```python
from build123d import *

# Parameters (mm, degrees)
SKETCH1_W           = 63.5
SKETCH1_H           = 50.8
BOSS_EXTRUDE1_DEPTH = 25.2
SKETCH2_R           = 13.1445
SKETCH2_R_2         = 6.7945
BOSS_EXTRUDE2_DEPTH = 2.2
SKETCH3_R           = 2
CUT_EXTRUDE1_DEPTH  = 5.5
SKETCH4_R           = 2
CUT_EXTRUDE2_DEPTH  = 5.5
CUT_EXTRUDE3_START  = -5.5
SKETCH5_R           = 2
CUT_EXTRUDE3_DEPTH  = 5.5
FILLET1_R           = 2
SKETCH6_W           = 18
SKETCH6_H           = 12
BOSS_EXTRUDE3_DEPTH = 1


with BuildPart() as part:
    # Sketch1 → Boss-Extrude1 (new body)
    with BuildSketch(Plane(origin=(0, 0, 0), x_dir=(1, 0, 0), z_dir=(0, 1, 0))):
        Rectangle(SKETCH1_W, SKETCH1_H)
    extrude(amount=BOSS_EXTRUDE1_DEPTH)

    # Sketch2 → Boss-Extrude2 (add)
    with BuildSketch(Plane(origin=(0, 25.2, 0), x_dir=(1, 0, 0), z_dir=(0, 1, 0))):
        with Locations(Location((15.25, 0, 0), (0, 0, 90))):
            Circle(SKETCH2_R)
        with Locations(Location((15.25, 0, 0), (0, 0, 270))):
            Circle(SKETCH2_R_2, mode=Mode.SUBTRACT)
    extrude(amount=BOSS_EXTRUDE2_DEPTH)

    # Sketch3 → Cut-Extrude1 (cut)
    with BuildSketch(Plane.XY.offset(25.4)):
        with Locations((15.25, 12.6)):
            Circle(SKETCH3_R)
    extrude(amount=-CUT_EXTRUDE1_DEPTH, mode=Mode.SUBTRACT)

    # Sketch4 → Cut-Extrude2 (cut)
    with BuildSketch(Plane(origin=(31.75, 0, 0), x_dir=(0, 0, -1), z_dir=(1, 0, 0))):
        with Locations((0, 12.6)):
            Circle(SKETCH4_R)
    extrude(amount=-CUT_EXTRUDE2_DEPTH, mode=Mode.SUBTRACT)

    # Sketch5 → Cut-Extrude3 (cut)
    with BuildSketch(Plane(origin=(0, 0, -25.4), x_dir=(-1, 0, 0), z_dir=(0, 0, -1)).offset(CUT_EXTRUDE3_START)):
        with Locations(Location((-15.25, 12.6, 0), (0, 0, 180))):
            Circle(SKETCH5_R)
    extrude(amount=CUT_EXTRUDE3_DEPTH, mode=Mode.SUBTRACT)

    # Fillet1
    fillet1_edges = [part.edges().sort_by_distance(p)[0] for p in [
        (-31.75, 25.2, 0),
        (0, 25.2, 25.4),
        (31.75, 25.2, 0),
        (0, 0, 25.4),
        (-31.75, 0, 0),
        (0, 0, -25.4),
        (31.75, 0, 0),
        (0, 25.2, -25.4),
        (31.75, 12.6, 25.4),
        (-31.75, 12.6, 25.4),
        (-31.75, 12.6, -25.4),
        (31.75, 12.6, -25.4),
    ]]
    fillet(fillet1_edges, radius=FILLET1_R)

    # Sketch6 → Boss-Extrude3 (add)
    with BuildSketch(Plane(origin=(0, 0, -25.4), x_dir=(-1, 0, 0), z_dir=(0, 0, -1))):
        with Locations((16.25, 8.5)):
            Rectangle(SKETCH6_W, SKETCH6_H)
    extrude(amount=BOSS_EXTRUDE3_DEPTH)


solid = part.part
```
Part model, mm, in its own coordinate system. A direction names the side the tool comes from. Coordinates: 2 decimals unless noted, no trailing zeros. Order: outer loops, then holes, each group sorted by start corner. A loop starts at its lowest first (then second) coordinate and runs counter-clockwise, first axis right, second up. Notation, with made-up numbers: (-23.5, -31.5) - (10.5, -31.5) arc R11 cw to (10.5, -27.5) - close; hole circle Ø6 at (64, 25). An arc over 180 degrees is marked (long way). Return JSON: item names as keys, results as strings. Group by question number.
Item 1: Cut at D-D (x = -12). List the corners of the cut face in (y, z).
Item 2: Pull direction Y, two halves, no side cores. Call faces 1 (the face through (31.15, 12.75, 24.83)), 2 (the face through (0.42, 0.6, 24.83)), 3 (the face through (14.99, 14.583, 22.688)): pulls with the +Y half, pulls with the -Y half, needs draft (parallel to the pull), parting line crosses it, or undercut.
Item 3: Which spindle directions (+Z, -Z, +X, -X, +Y, -Y) get a long thin tool onto all of the face, cutting with end or side? Do faces 4 (the face through (15, 13, 19.9)), 5 (the face through (2.217, 26.285, 1.711)), 6 (the face through (15, 13, -19.9)). Say none if no direction does.
Item 4: Cut at B-B (y = 12.6). List the corners of the cut face in (x, z).
Item 5: Cut at C-C (z = 14). List the corners of the cut face in (x, y).
Item 6: Cut at A-A (z = -21). List the corners of the cut face in (x, y).
Item 7: Pin check, flat tips, straight feed: pin 1 (4 mm diameter, centred on x = -4.5, y = 22.5, fed in from -Z); pin 2 (0.5 mm diameter, centred on x = -20, z = -26, fed in from -Y); pin 3 (1.1 mm diameter, centred on y = 7, z = -26, fed in from -X). Stop position of each tip, or through.
Item 8: Drill centre lines: probe 1 along Y at (x, z) = (15, -21); probe 2 along X at (y, z) = (26, 0); probe 3 along Y at (x, z) = (-27, 1.5). Where is each one in solid material? Low to high. Write a range as from..to.
Check values:
{
 "1": {"outline": "(0, -23.4) arc R2 ccw to (2, -25.4) - (2.5, -25.4) - (2.5, -26.4) - (14.5, -26.4) - (14.5, -25.4) - (23.2, -25.4) arc R2 ccw to (25.2, -23.4) - (25.2, 23.4) arc R2 ccw to (23.2, 25.4) - (2, 25.4) arc R2 ccw to (0, 23.4) - close"},
 "2": {"face 1": "needs draft", "face 2": "pulls with the -Y half", "face 3": "undercut"},
 "3": {"face 4": "+Z", "face 5": "+Y", "face 6": "-Z"},
 "4": {"outline": "(-31.75, -23.4) arc R2 ccw to (-29.75, -25.4) - (-25.25, -25.4) - (-25.25, -26.4) - (-7.25, -26.4) - (-7.25, -25.4) - (13.25, -25.4) - (13.25, -19.9) - (17.25, -19.9) - (17.25, -25.4) - (29.75, -25.4) arc R2 ccw to (31.75, -23.4) - (31.75, -2) - (26.25, -2) - (26.25, 2) - (31.75, 2) - (31.75, 23.4) arc R2 ccw to (29.75, 25.4) - (17.25, 25.4) - (17.25, 19.9) - (13.25, 19.9) - (13.25, 25.4) - (-29.75, 25.4) arc R2 ccw to (-31.75, 23.4) - close"},
 "5": {"outline": "(-31.75, 2) arc R2 ccw to (-29.75, 0) - (29.75, 0) arc R2 ccw to (31.75, 2) - (31.75, 23.2) arc R2 ccw to (29.75, 25.2) - (-29.75, 25.2) arc R2 ccw to (-31.75, 23.2) - close"},
 "6": {"outline": "(-31.75, 2) arc R2 ccw to (-29.75, 0) - (29.75, 0) arc R2 ccw to (31.75, 2) - (31.75, 23.2) arc R2 ccw to (29.75, 25.2) - (-29.75, 25.2) arc R2 ccw to (-31.75, 23.2) - close; hole circle Ø4 at (15.25, 12.6)"},
 "7": {"pin 1": "stops at z = -25.4", "pin 2": "stops at y = 2.5", "pin 3": "stops at x = -25.25"},
 "8": {"probe 1": "y = 0..10.62, 14.58..25.2", "probe 2": "x = 2.11..8.46, 22.04..28.39", "probe 3": "y = 0..25.2"}
}
